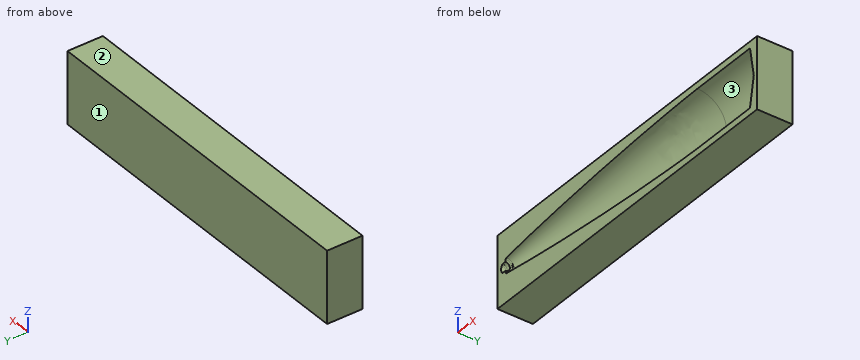
from build123d import *

# Parameters (mm, degrees)
REVOLVE1_ANGLE      = 180
SKETCH5_W           = 1002.922685695
SKETCH5_H           = 205.74
BOSS_EXTRUDE1_DEPTH = 38.1
SKETCH9_W           = 1002.922685695
SKETCH9_H           = 205.74
BOSS_EXTRUDE5_DEPTH = 101.6
FILLET1_R           = 3.175


with BuildPart() as part:
    # Sketch4 → Revolve1 (revolve)
    with BuildSketch(Plane(origin=(0, 0, 0), x_dir=(1, 0, 0), z_dir=(0, 1, 0))):
        with BuildLine():
            Line((838.2, 83.82), (1041.4, 83.82))
            Line((1041.4, 83.82), (1056.179727523, 0))
            Line((1056.179727523, 0), (78.657041828, 0))
            Line((78.657041828, 0), (83.91755407, 12.7))
            Line((83.91755407, 12.7), (96.61755407, 12.7))
            Line((96.61755407, 12.7), (98.163568293, 21.467882356))
            add(Edge.make_bspline(
                [(98.163568293, 21.467882356), (104.607343896, 22.497734344), (123.856103977, 25.493761031), (155.955742042, 30.152377402), (200.954778344, 36.105690484), (252.401123307, 42.315924819), (303.903852309, 48.038821007), (355.451699359, 53.337793152), (407.03781513, 58.250071041), (458.657158448, 62.799072617), (510.306365901, 66.995530477), (561.982906562, 70.840728542), (613.685068308, 74.325147511), (665.411655565, 77.427095788), (710.693213075, 79.771298327), (749.520698447, 81.471395458), (780.831665683, 82.597974895), (801.90983421, 83.214282129), (819.226060023, 83.601016067), (830.067936093, 83.761922773), (835.489248784, 83.813260117), (838.2, 83.82)],
                knots=[0.119382499, 0.119382499, 0.119382499, 0.119382499, 0.119382499, 0.150314205, 0.211721038, 0.273127872, 0.334534706, 0.395941541, 0.457348376, 0.518755211, 0.580162046, 0.641568881, 0.702975716, 0.764382551, 0.825789386, 0.887196222, 0.917899639, 0.948603057, 0.974301528, 0.987150764, 1, 1, 1, 1, 1], degree=4))
        make_face()
    revolve(axis=Axis((0, 0, 0), (1, 0, 0)), revolution_arc=REVOLVE1_ANGLE)

    # Sketch5 → Boss-Extrude1 (add)
    with BuildSketch(Plane.XZ):
        with Locations((567.418384676, 0)):
            Rectangle(SKETCH5_W, SKETCH5_H)
    extrude(amount=BOSS_EXTRUDE1_DEPTH)


with BuildPart() as body_2:
    # Sketch9 → Boss-Extrude5 (new body)
    with BuildSketch(Plane(origin=(0, 0, 0), x_dir=(1, 0, 0), z_dir=(0, 1, 0))):
        with Locations((567.418384676, 0)):
            Rectangle(SKETCH9_W, SKETCH9_H)
    extrude(amount=BOSS_EXTRUDE5_DEPTH)

    # Combine1: cut part
    add(part.part, mode=Mode.SUBTRACT)

    # Fillet1
    fillet1_edges = [body_2.edges().sort_by_distance(p)[0] for p in [
        (1041.4, 83.82, 0),
        (98.163568293, 21.467882356, 0),
        (83.91755407, 12.7, 0),
    ]]
    fillet(fillet1_edges, radius=FILLET1_R)


solid = body_2.part
Design review of the part built by this model. Coordinates are the model's own, in mm. Face numbers are marked on the shaded views. Coordinates: 2 decimals unless noted, no trailing zeros. Loops run counter-clockwise (first coordinate to the right, second up) from the corner with the lowest first, then second, coordinate; pieces in that order, holes last.
Item 1: Add section A-A (x = 908). Write out the cut boundary in (y, z), and give its area (3 significant figures).
Completed:
outline: (0, -102.87) - (101.6, -102.87) - (101.6, 102.87) - (0, 102.87) - (0, 83.82) arc R83.82 cw to (0, -83.82) - close
area: 9,870 mm2
Item 2: Wall thickness on L1, parallel to Z at x = 862, y = 59; L2, parallel to Z at x = 833.5, y = 30; L3, parallel to X at y = 8, z = 16: over which ranges is each line inside the solid? List them lowest first.
Completed:
L1: z = -102.87 to -59.54, 59.54 to 102.87
L2: z = -102.87 to -78.24, 78.24 to 102.87
L3: x = 65.96 to 97.53, 1053.03 to 1068.88
Item 3: Draft analysis for pull direction Z (two halves, no side actions). For the marked faces 1, 2 and 3, state which applies: pulls with the +Z half, pulls with the -Z half, needs draft (parallel to the pull), parting line crosses it, or undercut.
Completed:
face 1: needs draft
face 2: pulls with the +Z half
face 3: undercut
